Work out the finished part from the listing and answer in its coordinate system (mm). Coordinates: 2 decimals unless noted, no trailing zeros. Order: outer loops, then holes, each group sorted by start corner. A loop starts at its lowest first (then second) coordinate and runs counter-clockwise, first axis right, second up. Notation, with made-up numbers: M -36,76.25 L -30,76.25 A34 ccw -30,111.25 Z; hole C 60.5,67.25 d6. An arc over 180 degrees is marked long. Use a Markdown table: item, result. Add a question column.
from build123d import *

# Parameters (mm, degrees)
BOSS_EXTRUDE1_DEPTH = 10


with BuildPart() as part:
    # Sketch1 → Boss-Extrude1 (new body)
    with BuildSketch(Plane.XY):
        with BuildLine():
            Line((-78.611020919, 52.384922135), (126.388979081, -31.522054609))
            ThreePointArc((126.388979081, -31.522054609), (128.646483258, -33.362872526), (129.494976829, -36.149446474))
            Line((129.494976829, -36.149446474), (129.494976829, -44.793346711))
            ThreePointArc((129.494976829, -44.793346711), (128.030510735, -48.328880617), (124.494976829, -49.793346711))
            Line((124.494976829, -49.793346711), (-85.505023171, -49.793346711))
            Line((-85.505023171, -49.793346711), (-85.505023171, 47.75753027))
            ThreePointArc((-85.505023171, 47.75753027), (-83.29159712, 51.909036699), (-78.611020919, 52.384922135))
        make_face()
    extrude(amount=BOSS_EXTRUDE1_DEPTH)


solid = part.part
(1) A cutting plane is placed at C-C on y = 28. Write down the section's boundary in (x, z).
(2) A cutting plane is placed at B-B on x = -59. Write down the section's boundary in (y, z).
(3) Straight lines are drawn through the part: line 1 (X direction, y = -35.5, z = 7); line 2 (Y direction, x = 75, z = 9); line 3 (X direction, y = -4, z = 1.75). For each, find the intervals that lie inside material, in ascending order.
(4) A cutting plane is placed at A-A on z = 5.75. Write down the section's boundary in (x, y).
(5) Given P1, Ø2, axis at x = 73, z = 5.5, coming from the +Y side; P2, Ø4, axis at x = 45.5, y = 4, coming from the -Z side; P3, Ø4, axis at y = -26.5, z = 7.5, coming from the +X side; P4, Ø5, axis at y = 30, z = 6, coming from the +X side, each flat-ended and moving along its own axis, determine where each tip first touches the part or whether it passes through.
From the geometry:
| question | item | result |
|---|---|---|
| 1 | outline | M -85.51,0 L -19.03,0 L -19.03,10 L -85.51,10 Z |
| 2 | outline | M -49.79,0 L 44.36,0 L 44.36,10 L -49.79,10 Z |
| 3 | line 1 | x = -85.51 to 129.45 |
| 3 | line 2 | y = -49.79 to -10.49 |
| 3 | line 3 | x = -85.51 to 59.15 |
| 4 | outline | M -85.51,-49.79 L 124.49,-49.79 A5 ccw 129.49,-44.79 L 129.49,-36.15 A5 ccw 126.39,-31.52 L -78.61,52.38 A5 ccw -85.51,47.76 Z |
| 5 | P1 | stops at y = -9.26 |
| 5 | P2 | passes through |
| 5 | P3 | stops at x = 119.01 |
| 5 | P4 | stops at x = -17.81 |
